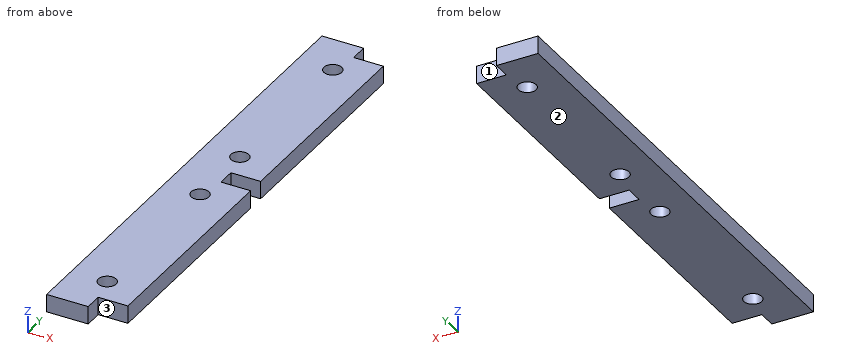
```python
from build123d import *

# Parameters (mm, degrees)
ESQUISSE1_R             = 1.5
BOSS_EXTRU_1_DEPTH      = 3
ESQUISSE2_W             = 12
ESQUISSE2_H             = 17.5
ENL_V_MAT_EXTRU_1_DEPTH = 119.190524155


with BuildPart() as part:
    # Esquisse1 → Boss.-Extru.1 (new body)
    with BuildSketch(Plane.XY):
        Polygon((-6, 0), (6, 0), (6, 17.5), (1, 17.5), (1, 20.5), (6, 20.5), (6, 57.5), (1, 57.5), (1, 60.5), (6, 60.5), (6, 97.5), (1, 97.5), (1, 100.5), (6, 100.5), (6, 118), (-6, 118), align=None)
        with Locations((0, 105)):
            Circle(ESQUISSE1_R, mode=Mode.SUBTRACT)
        with Locations(Location((0, 93, 0), (0, 0, 180))):
            Circle(ESQUISSE1_R, mode=Mode.SUBTRACT)
        with Locations((0, 65)):
            Circle(ESQUISSE1_R, mode=Mode.SUBTRACT)
        with Locations(Location((0, 53, 0), (0, 0, 180))):
            Circle(ESQUISSE1_R, mode=Mode.SUBTRACT)
        with Locations((0, 25)):
            Circle(ESQUISSE1_R, mode=Mode.SUBTRACT)
        with Locations(Location((0, 13, 0), (0, 0, 180))):
            Circle(ESQUISSE1_R, mode=Mode.SUBTRACT)
    extrude(amount=BOSS_EXTRU_1_DEPTH)

    # Esquisse2 → Enlèv. mat.-Extru.1 (cut, through all)
    with BuildSketch(Plane.XY.offset(3)):
        with Locations((0, 109.25)):
            Rectangle(ESQUISSE2_W, ESQUISSE2_H)
        with Locations((0, 8.75)):
            Rectangle(ESQUISSE2_W, ESQUISSE2_H)
    extrude(amount=-ENL_V_MAT_EXTRU_1_DEPTH, mode=Mode.SUBTRACT)


solid = part.part
```
CAD build for the part. Positions are in the model's coordinates, mm. Face numbers are marked on the shaded views. A direction names the side the tool comes from. Coordinates: 2 decimals unless noted, no trailing zeros. Order: outer loops, then holes, each group sorted by start corner. A loop starts at its lowest first (then second) coordinate and runs counter-clockwise, first axis right, second up. Notation, with made-up numbers: (71, 54) - (125, 54) arc R12 ccw to (125, 77) - close; hole circle Ø4 at (59, -13). An arc over 180 degrees is marked (long way). Use a Markdown table: item, result. Add a question column.
(1) Flat gauge pins, fed straight in: pin 1 (1.5 mm diameter, centred on x = 3.5, z = 2, fed in from +Y); pin 2 (1.5 mm diameter, centred on x = 4, z = 1, fed in from -Y); pin 3 (0.9 mm diameter, centred on y = 59.5, z = 1.5, fed in from +X); pin 4 (2.5 mm diameter, centred on x = 0, y = 65, fed in from -Z). Where does each tip first touch, or does it go through?
(2) Saw through at A-A (x = 0). Give the cut face in (y, z).
(3) Saw through at C-C (z = 1.35). Give the cut face in (x, y).
(4) Saw through at B-B (y = 25). Give the cut face in (x, z).
(5) Which spindle directions (+Z, -Z, +X, -X, +Y, -Y) get a long thin tool onto all of the face, cutting with end or side? Do the marked faces 1, 2 and 3. Say none if no direction does.
(6) Drill centre lines: line 1 along Y through (x, z) = (0, 1.65); line 2 along Y through (x, z) = (-0.75, 1.4); line 3 along Y through (x, z) = (3.25, 0.95). Where is each one in solid material? Low to high. Write a range as [from, to].
Solved:
| question | item | result |
|---|---|---|
| 1 | pin 1 | stops at y = 97.5 |
| 1 | pin 2 | stops at y = 20.5 |
| 1 | pin 3 | stops at x = 1 |
| 1 | pin 4 | passes through |
| 2 | outline | (17.5, 0) - (23.5, 0) - (23.5, 3) - (17.5, 3) - close; (26.5, 0) - (51.5, 0) - (51.5, 3) - (26.5, 3) - close; (54.5, 0) - (63.5, 0) - (63.5, 3) - (54.5, 3) - close; (66.5, 0) - (91.5, 0) - (91.5, 3) - (66.5, 3) - close; (94.5, 0) - (100.5, 0) - (100.5, 3) - (94.5, 3) - close |
| 3 | outline | (-6, 17.5) - (1, 17.5) - (1, 20.5) - (6, 20.5) - (6, 57.5) - (1, 57.5) - (1, 60.5) - (6, 60.5) - (6, 97.5) - (1, 97.5) - (1, 100.5) - (-6, 100.5) - close; hole circle Ø3 at (0, 25); hole circle Ø3 at (0, 53); hole circle Ø3 at (0, 65); hole circle Ø3 at (0, 93) |
| 4 | outline | (-6, 0) - (-1.5, 0) - (-1.5, 3) - (-6, 3) - close; (1.5, 0) - (6, 0) - (6, 3) - (1.5, 3) - close |
| 5 | face 1 | +Z, -Z, +X, +Y |
| 5 | face 2 | -Z, +X, -X, +Y, -Y |
| 5 | face 3 | +Z, -Z, +X, -Y |
| 6 | line 1 | y = [17.5, 23.5], [26.5, 51.5], [54.5, 63.5], [66.5, 91.5], [94.5, 100.5] |
| 6 | line 2 | y = [17.5, 23.7], [26.3, 51.7], [54.3, 63.7], [66.3, 91.7], [94.3, 100.5] |
| 6 | line 3 | y = [20.5, 57.5], [60.5, 97.5] |
